Here's how the part is built. I have some questions about the finished solid (model axes, mm). A direction names the side the tool comes from. Round coordinates to 2 decimals unless told otherwise and drop trailing zeros. Order: outer loops, then holes, each group sorted by start corner. A loop starts at its lowest first (then second) coordinate and runs counter-clockwise, first axis right, second up. Notation, with made-up numbers: M 32.5,17 L 52.5,17 A22 cw 52.5,44 Z; hole C 28.25,47.25 d5. An arc over 180 degrees is marked long. Write item = value, one per line. Start each with the question number.
Item 1: I want a section at B-B, the plane z = 0. List the corners of the cut face in (x, y) for me.
Item 2: Please list where these lines run through material, in increasing order: L1, parallel to X at y = 8.5, z = -14; L2, parallel to Z at x = 0, y = 3.05; L3, parallel to Z at x = 71.5, y = 9.75.
Item 3: I want a section at D-D, the plane z = 91. List the corners of the cut face in (x, y) for me.
Item 4: I want a section at C-C, the plane y = 3.25. List the corners of the cut face in (x, z) for me.
Item 5: For faces 4 (the face through (-91, 8, 27.725)), 5 (the face through (-78.1, 2.54, -17.34)), 6 (the face through (-67.191, 8, -4)), 7 (the face through (-31.808, 8, -90)), 8 (the face through (86, 8, 26.284)), which set-ups out of +Z, -Z, +X, -X, +Y, -Y let a thin tool reach every point of the face, with its end or its side?
Item 6: We'd pull the mould along Z, two halves only. Please class faces 1 (the face through (-1, 5, 71)), 2 (the face through (-2, 11, -68)), 3 (the face through (86, 8, -37.716)): pulls with the +Z half, pulls with the -Z half, needs draft (parallel to the pull), parting line crosses it, or undercut.
Item 7: I'm going to push flat-ended pins straight in: P1, Ø2.5, axis at y = 9.5, z = 88.5, coming from the +X side; P2, Ø2.5, axis at x = 89.5, y = 9.5, coming from the +Z side; P3, Ø6, axis at x = 21, z = -66.5, coming from the -Y side; P4, Ø10, axis at x = -60, z = 43.5, coming from the +Y side. Where does each tip first touch, or does it pass through?
Item 8: I want a section at A-A, the plane x = 0. List the corners of the cut face in (y, z) for me.
```python
from build123d import *

# Parameters (mm, degrees)
SKETCH_1_R          = 100
EXTRUDE_2_DEPTH     = 5
SKETCH_3_R          = 80
CUT_EXTRUDE_1_DEPTH = 5
SKETCH_4_W          = 64
SKETCH_4_H          = 47
SKETCH_4_W_2        = 47
SKETCH_4_H_2        = 64
EXTRUDE_4_DEPTH     = 6
SKETCH_7_W          = 60
SKETCH_7_H          = 43
SKETCH_7_W_2        = 43
SKETCH_7_H_2        = 60
CUT_EXTRUDE_2_DEPTH = 3


with BuildPart() as part:
    # 草图1 → 凸台-拉伸2 (new body)
    with BuildSketch(Plane(origin=(0, 0, 0), x_dir=(1, 0, 0), z_dir=(0, 1, 0))):
        with Locations(Location((0, 0, 0), (0, 0, 270))):
            Circle(SKETCH_1_R)
    extrude(amount=EXTRUDE_2_DEPTH)

    # 草图3 → 切除-拉伸1 (cut)
    with BuildSketch(Plane(origin=(0, 5, 0), x_dir=(1, 0, 0), z_dir=(0, 1, 0))):
        with Locations(Location((0, 0, 0), (0, 0, 270))):
            Circle(SKETCH_3_R)
    extrude(amount=-CUT_EXTRUDE_1_DEPTH, mode=Mode.SUBTRACT)

    # 草图4 → 凸台-拉伸4 (add)
    with BuildSketch(Plane(origin=(0, 5, 0), x_dir=(1, 0, 0), z_dir=(0, 1, 0))):
        with Locations((-0.162859843, -88.550006354)):
            Rectangle(SKETCH_4_W, SKETCH_4_H)
        with Locations((0.19173376, 90.641323137)):
            Rectangle(SKETCH_4_W, SKETCH_4_H)
        with Locations((-90.690666059, 4.275289792)):
            Rectangle(SKETCH_4_W_2, SKETCH_4_H_2)
        with Locations((86.540113404, 5.715544521)):
            Rectangle(SKETCH_4_W_2, SKETCH_4_H_2)
    extrude(amount=EXTRUDE_4_DEPTH)

    # 草图7 → 切除-拉伸2 (cut)
    with BuildSketch(Plane(origin=(0, 11, 0), x_dir=(1, 0, 0), z_dir=(0, 1, 0))):
        with Locations((-0.461103179, -88.439082163)):
            Rectangle(SKETCH_7_W, SKETCH_7_H)
        with Locations((0.274660962, 90.782811556)):
            Rectangle(SKETCH_7_W, SKETCH_7_H)
        with Locations((86.697399142, 5.490846131)):
            Rectangle(SKETCH_7_W_2, SKETCH_7_H_2)
        with Locations((-90.460833893, 4.260878525)):
            Rectangle(SKETCH_7_W_2, SKETCH_7_H_2)
    extrude(amount=-CUT_EXTRUDE_2_DEPTH, mode=Mode.SUBTRACT)


solid = part.part
```
Filled in:
q1.outline = M -114.19,5 L -100,5 L -100,0 L -80,0 L -80,5 L -67.19,5 L -67.19,11 L -68.96,11 L -68.96,8 L -111.96,8 L -111.96,11 L -114.19,11 Z; M 63.04,5 L 80,5 L 80,0 L 100,0 L 100,5 L 110.04,5 L 110.04,11 L 108.2,11 L 108.2,8 L 65.2,8 L 65.2,11 L 63.04,11 Z
q2.L1 = -114.19 to -111.96, -68.96 to -67.19, 63.04 to 65.2, 108.2 to 110.04
q2.L2 = -100 to -80, 80 to 100
q2.L3 = -37.72 to -35.49, 24.51 to 26.28
q3.outline = M -41.46,0 L 41.46,0 L 41.46,5 L 31.84,5 L 31.84,11 L 29.54,11 L 29.54,8 L -30.46,8 L -30.46,11 L -32.16,11 L -32.16,5 L -41.46,5 Z
q4.outline = C 0,0 d200; hole C 0,0 d160
q5.face_4 = +Z, +X, -X, +Y
q5.face_5 = -Y
q5.face_6 = +Z, -Z, +Y, -Y
q5.face_7 = -Z, -X, +Y
q5.face_8 = +Z, +X, +Y
q6.face_1 = undercut
q6.face_2 = needs draft
q6.face_3 = pulls with the -Z half
q7.P1 = 31.84
q7.P2 = 26.28
q7.P3 = 5
q7.P4 = through
q8.outline = M 0,-100 L 5,-100 L 5,-114.14 L 11,-114.14 L 11,-112.28 L 8,-112.28 L 8,-69.28 L 11,-69.28 L 11,-67.14 L 5,-67.14 L 5,-80 L 0,-80 Z; M 0,80 L 5,80 L 5,65.05 L 11,65.05 L 11,66.94 L 8,66.94 L 8,109.94 L 11,109.94 L 11,112.05 L 5,112.05 L 5,100 L 0,100 Z
